Read the model definition and answer for the solid it produces. Units are mm, in the model's axes. A direction names the side the tool comes from. Give positions to 0.01 mm unless a question says otherwise; leave off trailing zeros. Loops run counter-clockwise (first coordinate to the right, second up) from the corner with the lowest first, then second, coordinate; pieces in that order, holes last.
(1) Determine the mould class of faces 5 (the face through (10, 5, 5)), 6 (the face through (30, 20, 10)), 7 (the face through (29, 43, 10)) for opening direction Y: pulls with the +Y half, pulls with the -Y half, needs draft (parallel to the pull), parting line crosses it, or undercut.
(2) Straight lines are drawn through the part: probe 1 along X at (y, z) = (16, 16.25); probe 2 along Y at (x, z) = (19.25, 6.25); probe 3 along X at (y, z) = (30, 13.5). For each, find the intervals that lie inside material, in ascending order.
(3) This flat-tipped pin is pushed along its axis until it touches: P1, Ø3, axis at y = 5.5, z = 6, coming from the +X side. Where does it stop, or does it pass through?
(4) Find section A-A, the plane z = 14.5. Write down the section's boundary in (x, y).
(5) Find section B-B, the plane y = 11.5. Write down the section's boundary in (x, z), then the cut area to 3 significant figures.
(6) Find section D-D, the plane y = 5.25. Write down the section's boundary in (x, z).
(7) Find section C-C, the plane x = 21.25. Write down the section's boundary in (y, z), then the cut area to 3 significant figures.
(8) Which of the six approach directions +Z, -Z, +X, -X, +Y, -Y give full straight-line access (tool end or side, diameter ignored) to faces 1 (the face through (20.14, 8.35, 5.98)), 2 (the face through (15.4, 42.744, 15.07)), 3 (the face through (15, 0, 8)), 4 (the face through (25, 11, 15))?
```python
from build123d import *

# Parameters (mm, degrees)
F0_W     = 29.999999
F0_H     = 45
F1_DEPTH = 20
F2_R     = 12.75
F3_DEPTH = 10
F4_R     = 3.25
F5_DEPTH = 20
F6_W     = 20
F6_H     = 22.090354
F7_DEPTH = 10
F8_R     = 5


with BuildPart() as f1:
    # F0 (on Top) → F1 (new body)
    with BuildSketch(Plane.XY):
        with Locations((14.999999, 22.5)):
            Rectangle(F0_W, F0_H)
    extrude(amount=F1_DEPTH)

    # F2 (on face) → F3 (cut)
    with BuildSketch(Plane.XY.offset(20)):
        with Locations((14.999999, 30)):
            Circle(F2_R)
    extrude(amount=-F3_DEPTH, mode=Mode.SUBTRACT)

    # F4 (on face) → F5 (cut)
    with BuildSketch(Plane.YZ.offset(29.999999)):
        with Locations((5.25, 5)):
            Circle(F4_R)
    extrude(amount=-F5_DEPTH, mode=Mode.SUBTRACT)

    # F6 (on face) → F7 (cut)
    with BuildSketch(Plane.XY.offset(20)):
        with Locations((14.999999, 11.045177)):
            Rectangle(F6_W, F6_H)
    extrude(amount=-F7_DEPTH, mode=Mode.SUBTRACT)

    # F8
    f8_edges = [f1.edges().sort_by_distance(p)[0] for p in [
        (0, 45, 10),
        (29.999999, 45, 10),
    ]]
    fillet(f8_edges, radius=F8_R)


solid = f1.part
```
Entries:
1. face 5: undercut
1. face 6: needs draft
1. face 7: pulls with the +Y half
2. probe 1: x = 0 to 5, 25 to 30
2. probe 2: y = 0 to 2.25, 8.25 to 45
2. probe 3: x = 0 to 2.25, 27.75 to 30
3. P1: stops at x = 10
4. outline: (0, 0) - (5, 0) - (5, 22.09) arc R12.75 cw (long way) to (25, 22.09) - (25, 0) - (30, 0) - (30, 40) arc R5 ccw to (25, 45) - (5, 45) arc R5 ccw to (0, 40) - close
5. outline: (0, 0) - (30, 0) - (30, 20) - (25, 20) - (25, 10) - (5, 10) - (5, 20) - (0, 20) - close
5. area: 400 mm2
6. outline: (0, 0) - (30, 0) - (30, 1.75) - (10, 1.75) - (10, 8.25) - (30, 8.25) - (30, 20) - (25, 20) - (25, 10) - (5, 10) - (5, 20) - (0, 20) - close
7. outline: (0, 0) - (45, 0) - (45, 20) - (41.11, 20) - (41.11, 10) - (0, 10) - close; hole circle Ø6.5 at (5.25, 5)
7. area: 456 mm2
8. face 1: +X
8. face 2: +Z
8. face 3: +Z, -Z, +X, -X, -Y
8. face 4: +Z, -Y
